```python
from build123d import *

# Parameters (mm, degrees)
F0_W          = 10
F0_H          = 40
F1_DEPTH      = 30
F1_DEPTH_BACK = 30
F2_R          = 1
F3_DEPTH      = 4
F4_DEPTH      = 15


with BuildPart() as f1:
    # F0 (on Right) → F1 (new body, two sides)
    with BuildSketch(Plane.YZ) as f1_sk:
        Rectangle(F0_W, F0_H)
    extrude(amount=F1_DEPTH)
    extrude(f1_sk.sketch, amount=-F1_DEPTH_BACK)

    # F2 (on face) → F3 (join)
    with BuildSketch(Plane.XZ.offset(5)):
        with Locations((-18, 14)):
            Circle(F2_R)
        with Locations((-18, -12)):
            Circle(F2_R)
        with Locations((7, -12)):
            Circle(F2_R)
    extrude(amount=F3_DEPTH)

    # F4 (add): a face of the model
    f4_faces = [f1.faces().sort_by_distance(p)[0] for p in [
        (0, 0, 20),
    ]]
    extrude(f4_faces, amount=F4_DEPTH)


solid = f1.part
```
The listing builds one solid part. Answer for the finished solid, in the listing's coordinates (mm). A direction names the side the tool comes from. Give positions to 0.01 mm unless a question says otherwise; leave off trailing zeros. Order: outer loops, then holes, each group sorted by start corner. A loop starts at its lowest first (then second) coordinate and runs counter-clockwise, first axis right, second up. Notation, with made-up numbers: (7, 0) -> (55, 0) arc R20 ccw to (55, 9) -> close; hole circle Ø6 at (-1.5, 13). An arc over 180 degrees is marked (long way). Answer as a JSON object with one key per item and string values. Group by question number.
Item 1: A flat-ended cylindrical pin translates along its axis: pin 1 (6 mm diameter, centred on x = 6.5, z = 0.5, fed in from -Y). Find the tip coordinate at first contact, or state that the pin passes through.
Item 2: Determine the mould class of faces 3 (the flat face through (7, -9, -12)), 4 (the flat face through (0, 0, 35)), 5 (the cylindrical face through (-18, -7, 13)) for opening direction Z: pulls with the +Z half, pulls with the -Z half, needs draft (parallel to the pull), parting line crosses it, or undercut.
Item 3: The part is cut by section A-A on x = 7. Write down the section's boundary in (y, z), and give its area (3 significant figures).
Item 4: The part is cut by section D-D on z = -12. Write down the section's boundary in (x, y).
Item 5: A tool of negligible diameter and unlimited length cuts with its end or side. For faces 1 (the flat face through (0, 5, 7)), 2 (the cylindrical face through (-18.737, -6.972, -11.324)), from which of +Z, -Z, +X, -X, +Y, -Y can it reach the whole face along a straight path? Write none if from no direction.
Item 6: Consider L1, parallel to Y at x = -3, z = -6.5. Determine where the line is inside the solid, lowest interval first. Write a range as from..to.
Item 7: The part is cut by section B-B on z = 14. Write down the section's boundary in (x, y).
Item 8: The part is cut by section C-C on y = -7.75. Write down the section's boundary in (x, z), and give its area (3 significant figures).
Result set:
{
 "1": {"pin 1": "y = -5"},
 "2": {"face 3": "needs draft", "face 4": "pulls with the +Z half", "face 5": "undercut"},
 "3": {"outline": "(-9, -13) -> (-5, -13) -> (-5, -20) -> (5, -20) -> (5, 35) -> (-5, 35) -> (-5, -11) -> (-9, -11) -> close", "area": "558 mm²"},
 "4": {"outline": "(-30, -5) -> (-19, -5) -> (-19, -9) -> (-17, -9) -> (-17, -5) -> (6, -5) -> (6, -9) -> (8, -9) -> (8, -5) -> (30, -5) -> (30, 5) -> (-30, 5) -> close"},
 "5": {"face 1": "+Z, -Z, +X, -X, +Y", "face 2": "-Y"},
 "6": {"L1": "-5..5"},
 "7": {"outline": "(-30, -5) -> (-19, -5) -> (-19, -9) -> (-17, -9) -> (-17, -5) -> (30, -5) -> (30, 5) -> (-30, 5) -> close"},
 "8": {"outline": "circle Ø2 at (-18, -12); circle Ø2 at (-18, 14); circle Ø2 at (7, -12)", "area": "9.42 mm²"}
}
